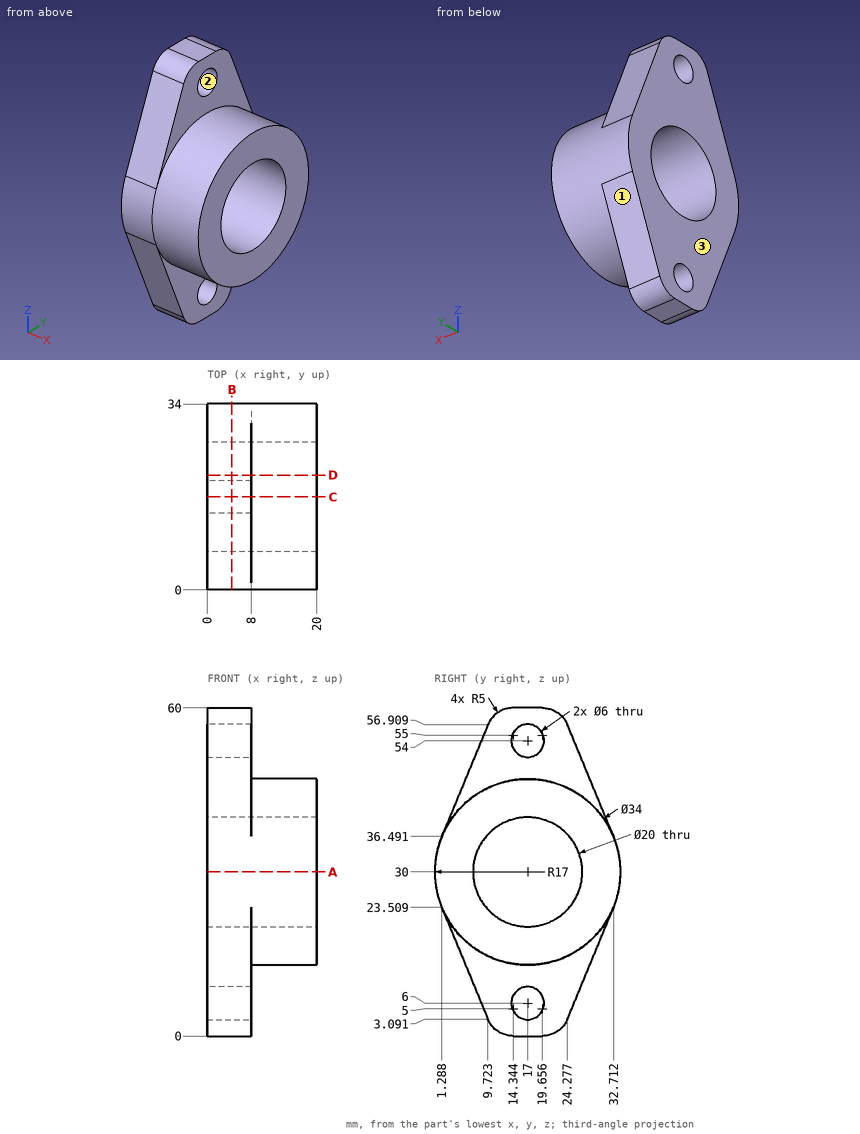
Answer from the drawing. Dimensions are ordinates in mm from the lowest x, y and z of the part. Coordinates: 2 decimals unless noted, no trailing zeros. Write each loop counter-clockwise with the first axis right and the second up, starting at its lowest first coordinate (ties: lowest second). Pieces come first, ordered by that corner, then holes. Notation, with made-up numbers: (-16.75, 75.25) - (13.25, 75.25) arc R8 ccw to (13.25, 80.25) - close; hole circle Ø3 at (46.25, 2.5). An arc over 180 degrees is marked (long way). Return JSON: item names as keys, results as strings.
1. Each of these flat-tipped pins is pushed along its axis until it touches: pin 1 Ø1 at (x, y) = (3, 25) entering from +Z; pin 2 Ø5 at (x, y) = (8.5, 11.5) entering from -Z; pin 3 Ø6 at (x, y) = (4.5, 6) entering from +Z. Where does it stop, or does it pass through?
Final values:
{"pin 1": "z = 56.37", "pin 2": "z = 0.02", "pin 3": "z = 55.16"}
2. For a pull along Z with two mould halves and no side action, classify the marked faces 1, 2 and 3 as +Z half, -Z half, draft (parallel to the pull), parting line (faces both ways), or undercut.
Final values:
{"face 1": "-Z half", "face 2": "undercut", "face 3": "draft"}
3. The part is cut by section B-B on x = 4.5. Determine the outline of the cut face in (y, z), then the cut area to 3 significant figures.
Final values:
{"outline": "(1.29, 23.51) - (9.72, 3.09) arc R5 ccw to (14.34, 0) - (19.66, 0) arc R5 ccw to (24.28, 3.09) - (32.71, 23.51) arc R17 ccw to (32.71, 36.49) - (24.28, 56.91) arc R5 ccw to (19.66, 60) - (14.34, 60) arc R5 ccw to (9.72, 56.91) - (1.29, 36.49) arc R17 ccw to start; hole circle Ø20 at (17, 30); hole circle Ø6 at (17, 6); hole circle Ø6 at (17, 54)", "area": "1,070 mm^2"}
4. The part is cut by section C-C on y = 17. Determine the outline of the cut face in (x, z).
Final values:
{"outline": "(0, 0) - (8, 0) - (8, 3) - (0, 3) - close; (0, 9) - (8, 9) - (8, 13) - (20, 13) - (20, 20) - (0, 20) - close; (0, 40) - (20, 40) - (20, 47) - (8, 47) - (8, 51) - (0, 51) - close; (0, 57) - (8, 57) - (8, 60) - (0, 60) - close"}
5. Consider line 1 along Y through (x, z) = (12.5, 30); line 2 along Z through (x, y) = (2.75, 16); line 3 along Z through (x, y) = (5.75, 24) (1 decimal). Determine where each line is inside the solid, lowest interval first.
Final values:
{"line 1": "0 to 7, 27 to 34", "line 2": "0 to 3.17, 8.83 to 20.05, 39.95 to 51.17, 56.83 to 60", "line 3": "2.5 to 22.9, 37.1 to 57.5"}
6. The part is cut by section A-A on z = 30. Determine the outline of the cut face in (x, y), then the cut area to 3 significant figures.
Final values:
{"outline": "(0, 0) - (20, 0) - (20, 7) - (0, 7) - close; (0, 27) - (20, 27) - (20, 34) - (0, 34) - close", "area": "280 mm^2"}
7. The part is cut by section D-D on y = 21. Determine the outline of the cut face in (x, z) (1 decimal), then the cut area to 3 significant figures.
Final values:
{"outline": "(0, 0.2) - (8, 0.2) - (8, 13.5) - (20, 13.5) - (20, 20.8) - (0, 20.8) - close; (0, 39.2) - (20, 39.2) - (20, 46.5) - (8, 46.5) - (8, 59.8) - (0, 59.8) - close", "area": "507 mm^2"}
